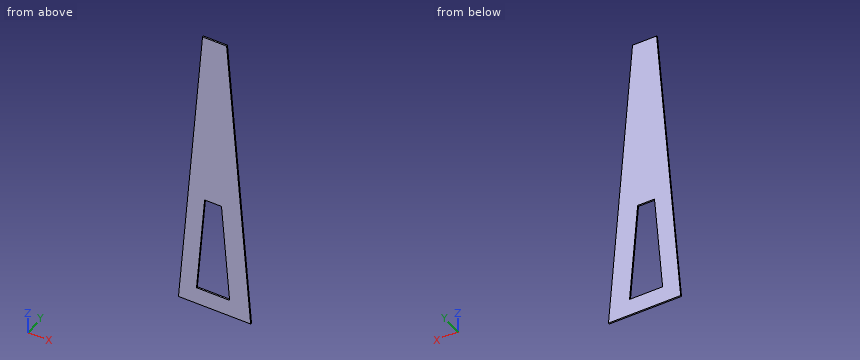
```python
from build123d import *

# Parameters (mm, degrees)
BOSS_EXTRUDE1_DEPTH = 1.524
CUT_EXTRUDE1_DEPTH  = 1.524


with BuildPart() as part:
    # Sketch1 → Boss-Extrude1 (new body)
    with BuildSketch(Plane(origin=(0, 0, 0), x_dir=(1, 0, 0), z_dir=(0, 1, 0))):
        Polygon((0, 0), (76.2, 0), (50.8, -314.706), (25.4, -314.706), align=None)
    extrude(amount=BOSS_EXTRUDE1_DEPTH)

    # Sketch4 → Cut-Extrude1 (cut)
    with BuildSketch(Plane(origin=(0, 0, 0), x_dir=(-1, 0, 0), z_dir=(0, -1, 0))):
        Polygon((-27.61263984, -124.689571655), (-45.39263984, -124.689571655), (-53.982012586, -18.267243325), (-19.023267093, -18.267243325), align=None)
    extrude(amount=-CUT_EXTRUDE1_DEPTH, mode=Mode.SUBTRACT)


solid = part.part
```
Build history of the part. All positions in model axes, mm. Round coordinates to 2 decimals unless told otherwise and drop trailing zeros. Loops run counter-clockwise (first coordinate to the right, second up) from the corner with the lowest first, then second, coordinate; pieces in that order, holes last.
Item 1: Saw through at B-B (y = 0.95). List the corners of the cut face in (x, z), then the cut area to 3 significant figures.
Item 2: Saw through at D-D (x = 65). List the corners of the cut face in (y, z).
Item 3: Saw through at C-C (z = 47). List the corners of the cut face in (x, y), then the cut area to 3 significant figures.
Item 4: Drill centre lines: line 1 along Z through (x, y) = (33.5, 1.15); line 2 along X through (y, z) = (0.6, 111); line 3 along X through (y, z) = (1.45, 56). Where is each one in solid material? Low to high.
Item 5: Saw through at A-A (x = 36). List the corners of the cut face in (y, z).
Worked answers:
1. outline: (0, 0) - (76.2, 0) - (50.8, 314.71) - (25.4, 314.71) - close; hole (19.02, 18.27) - (53.98, 18.27) - (45.39, 124.69) - (27.61, 124.69) - close
1. area: 13,200 mm2
2. outline: (0, 0) - (1.52, 0) - (1.52, 138.77) - (0, 138.77) - close
3. outline: (3.79, 0) - (21.34, 0) - (21.34, 1.52) - (3.79, 1.52) - close; (51.66, 0) - (72.41, 0) - (72.41, 1.52) - (51.66, 1.52) - close
3. area: 58.4 mm2
4. line 1: z = 0 to 18.27, 124.69 to 314.71
4. line 2: x = 8.96 to 26.51, 46.5 to 67.24
4. line 3: x = 4.52 to 22.07, 50.94 to 71.68
5. outline: (0, 0) - (1.52, 0) - (1.52, 18.27) - (0, 18.27) - close; (0, 124.69) - (1.52, 124.69) - (1.52, 314.71) - (0, 314.71) - close
